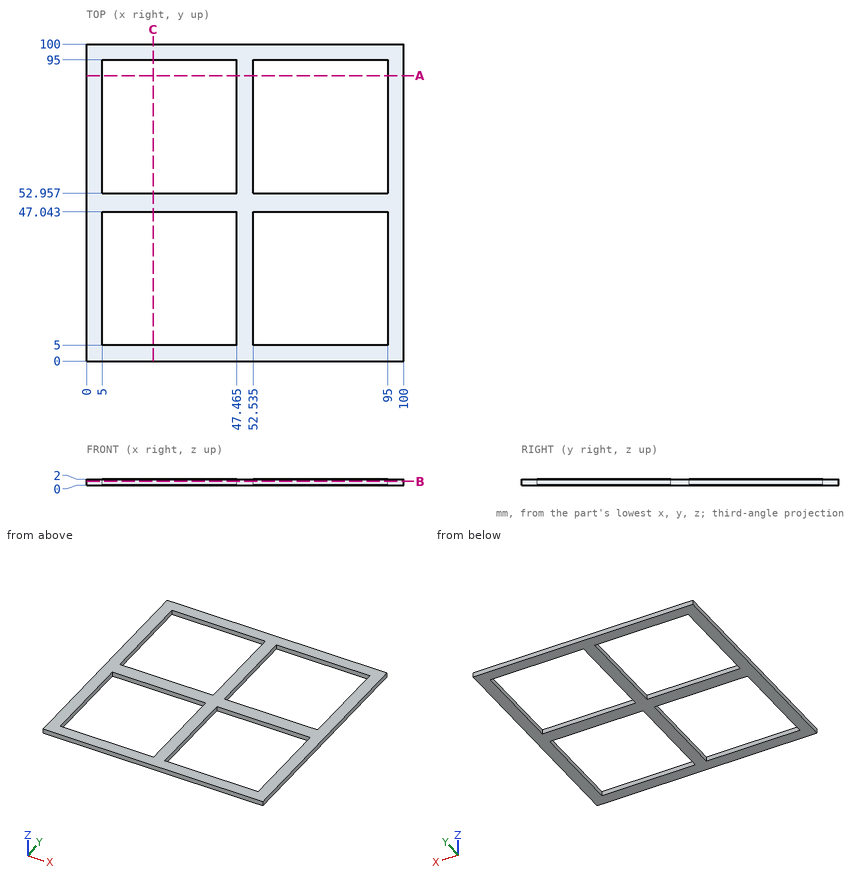
Check sheet for the drawn part. Datum: minimum x, y, z corner. Units: mm. Give positions to 0.01 mm unless a question says otherwise; leave off trailing zeros. Order: outer loops, then holes, each group sorted by start corner. A loop starts at its lowest first (then second) coordinate and runs counter-clockwise, first axis right, second up. Notation, with made-up numbers: (21, -11.75) -> (48, -11.75) arc R26 cw to (48, 4.25) -> close; hole circle Ø4 at (58, 85). An arc over 180 degrees is marked (long way). One line per item, written item: value.
(1) Sectioned sample at C-C on x = 21. Record the cut outline in (y, z).
Final values:
outline: (0, 0) -> (5, 0) -> (5, 2) -> (0, 2) -> close; (47.04, 0) -> (52.96, 0) -> (52.96, 2) -> (47.04, 2) -> close; (95, 0) -> (100, 0) -> (100, 2) -> (95, 2) -> close
(2) Sectioned sample at B-B on z = 1.25. Record the cut outline in (x, y) (1 decimal).
Final values:
outline: (0, 0) -> (100, 0) -> (100, 100) -> (0, 100) -> close; hole (5, 5) -> (47.5, 5) -> (47.5, 47) -> (5, 47) -> close; hole (5, 53) -> (47.5, 53) -> (47.5, 95) -> (5, 95) -> close; hole (52.5, 5) -> (95, 5) -> (95, 47) -> (52.5, 47) -> close; hole (52.5, 53) -> (95, 53) -> (95, 95) -> (52.5, 95) -> close
(3) Sectioned sample at A-A on y = 90. Record the cut outline in (x, z) (1 decimal).
Final values:
outline: (0, 0) -> (5, 0) -> (5, 2) -> (0, 2) -> close; (47.5, 0) -> (52.5, 0) -> (52.5, 2) -> (47.5, 2) -> close; (95, 0) -> (100, 0) -> (100, 2) -> (95, 2) -> close
(4) Scan lines: line 1 along Y through (x, z) = (72.5, 1.7); line 2 along X through (y, z) = (94, 0.85) (1 decimal). Record each from-to range of solid material in increasing order. Write a range as [from, to].
Final values:
line 1: [0, 5], [47.04, 52.96], [95, 100]
line 2: [0, 5], [47.5, 52.5], [95, 100]
